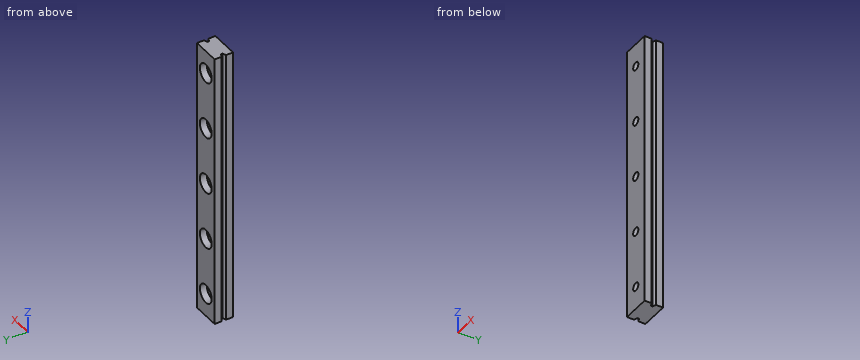
from build123d import *

# Parameters (mm, degrees)
SKETCH_1_W          = 12
SKETCH_1_H          = 8
EXTRUDE_1_DEPTH     = 120
SKETCH_2_R          = 1.75
CUT_EXTRUDE_1_DEPTH = 9
SKETCH_3_R          = 4
CUT_EXTRUDE_2_DEPTH = 3
CUT_EXTRUDE_3_DEPTH = 121


with BuildPart() as part:
    # 草图1 → 凸台-拉伸1 (new body)
    with BuildSketch(Plane.XY):
        Rectangle(SKETCH_1_W, SKETCH_1_H)
    extrude(amount=EXTRUDE_1_DEPTH)

    # 草图2 → 切除-拉伸1 (cut, through all)
    with BuildSketch(Plane(origin=(0, 4, 0), x_dir=(1, 0, 0), z_dir=(0, 1, 0))):
        with Locations((0, -10)):
            Circle(SKETCH_2_R)
        with Locations((0, -35)):
            Circle(SKETCH_2_R)
        with Locations((0, -60)):
            Circle(SKETCH_2_R)
        with Locations((0, -85)):
            Circle(SKETCH_2_R)
        with Locations((0, -110)):
            Circle(SKETCH_2_R)
        with Locations((0, -135)):
            Circle(SKETCH_2_R)
        with Locations((0, -160)):
            Circle(SKETCH_2_R)
        with Locations((0, -185)):
            Circle(SKETCH_2_R)
        with Locations((0, -210)):
            Circle(SKETCH_2_R)
        with Locations((0, -235)):
            Circle(SKETCH_2_R)
        with Locations((0, -260)):
            Circle(SKETCH_2_R)
        with Locations((0, -285)):
            Circle(SKETCH_2_R)
    extrude(amount=-CUT_EXTRUDE_1_DEPTH, mode=Mode.SUBTRACT)

    # 草图3 → 切除-拉伸2 (cut)
    with BuildSketch(Plane(origin=(0, 4, 0), x_dir=(1, 0, 0), z_dir=(0, 1, 0))):
        with Locations((0, -10)):
            Circle(SKETCH_3_R)
        with Locations((0, -35)):
            Circle(SKETCH_3_R)
        with Locations((0, -60)):
            Circle(SKETCH_3_R)
        with Locations((0, -85)):
            Circle(SKETCH_3_R)
        with Locations((0, -110)):
            Circle(SKETCH_3_R)
        with Locations((0, -135)):
            Circle(SKETCH_3_R)
        with Locations((0, -160)):
            Circle(SKETCH_3_R)
        with Locations((0, -185)):
            Circle(SKETCH_3_R)
        with Locations((0, -210)):
            Circle(SKETCH_3_R)
        with Locations((0, -235)):
            Circle(SKETCH_3_R)
        with Locations((0, -260)):
            Circle(SKETCH_3_R)
        with Locations((0, -285)):
            Circle(SKETCH_3_R)
    extrude(amount=-CUT_EXTRUDE_2_DEPTH, mode=Mode.SUBTRACT)

    # 草图4 → 切除-拉伸3 (cut, through all)
    with BuildSketch(Plane(origin=(0, 0, 0), x_dir=(-1, 0, 0), z_dir=(0, 0, -1))):
        Polygon((6, 1), (4.5, 0.3), (4.5, -0.3), (6, -1), align=None)
        Polygon((-6, 1), (-4.5, 0.3), (-4.5, -0.3), (-6, -1), align=None)
    extrude(amount=-CUT_EXTRUDE_3_DEPTH, mode=Mode.SUBTRACT)


solid = part.part
CAD build for the part. Positions are in the model's coordinates, mm. Round coordinates to 2 decimals unless told otherwise and drop trailing zeros. Write each loop counter-clockwise with the first axis right and the second up, starting at its lowest first coordinate (ties: lowest second). Pieces come first, ordered by that corner, then holes.
(1) Slice it at C-C, the plane z = 21. Write the cut outline in (x, y).
(2) Probe line 1 along Z through (x, y) = (0, 2.85); line 2 along Z through (x, y) = (0, -1.7); line 3 along X through (y, z) = (-1, 110). List the from-to ranges inside material, lowest first.
(3) Drop flat-ended pins along their axis: P1, Ø4, axis at x = 1, z = 86, coming from the +Y side; P2, Ø6.5, axis at x = 1.5, z = 11.5, coming from the +Y side. Give the stop position or say it passes through.
(4) Slice it at D-D, the plane x = 0. Count the separate pieces of the cut face and the enclosed holes in it, and give its area (4 significant figures).
(5) Slice it at A-A, the plane z = 35. Write the cut outline in (x, y).
(6) Slice it at B-B, the plane y = 2. Write the cut outline in (x, z).
From the geometry:
1. outline: (-6, -4) - (6, -4) - (6, -1) - (4.5, -0.3) - (4.5, 0.3) - (6, 1) - (6, 4) - (-6, 4) - (-6, 1) - (-4.5, 0.3) - (-4.5, -0.3) - (-6, -1) - close
2. line 1: z = 0 to 6, 14 to 31, 39 to 56, 64 to 81, 89 to 106, 114 to 120
2. line 2: z = 0 to 8.25, 11.75 to 33.25, 36.75 to 58.25, 61.75 to 83.25, 86.75 to 108.25, 111.75 to 120
2. line 3: x = -6 to -1.75, 1.75 to 6
3. P1: stops at y = 1
3. P2: stops at y = 4
4. separate pieces: 6
4. enclosed holes: 0
4. area: 752.5 mm2
5. outline: (-6, -4) - (-1.75, -4) - (-1.75, 1) - (-4, 1) - (-4, 4) - (-6, 4) - (-6, 1) - (-4.5, 0.3) - (-4.5, -0.3) - (-6, -1) - close; (1.75, -4) - (6, -4) - (6, -1) - (4.5, -0.3) - (4.5, 0.3) - (6, 1) - (6, 4) - (4, 4) - (4, 1) - (1.75, 1) - close
6. outline: (-6, 0) - (6, 0) - (6, 120) - (-6, 120) - close; hole circle Ø8 at (0, 10); hole circle Ø8 at (0, 35); hole circle Ø8 at (0, 60); hole circle Ø8 at (0, 85); hole circle Ø8 at (0, 110)
